Model file for the job. Use its own axes, mm. A direction names the side the tool comes from. Coordinates: 2 decimals unless noted, no trailing zeros. Order: outer loops, then holes, each group sorted by start corner. A loop starts at its lowest first (then second) coordinate and runs counter-clockwise, first axis right, second up. Notation, with made-up numbers: (26.5, -33) - (66.5, -33) arc R10 cw to (66.5, -29) - close; hole circle Ø5 at (-9, 47.25). An arc over 180 degrees is marked (long way). Put each result on its own line as item: value. Start each with the question number.
```python
from build123d import *

# Parameters (mm, degrees)
ESQUISSE1_R      = 5
EXTRUSION1_DEPTH = 3
ESQUISSE3_R      = 2
EXTRUSION3_DEPTH = 2
ESQUISSE4_R      = 5
EXTRUSION4_DEPTH = 1
ESQUISSE5_W      = 6
ESQUISSE5_H      = 12
EXTRUSION5_DEPTH = 10
ESQUISSE6_W      = 3
ESQUISSE6_H      = 2
EXTRUSION6_DEPTH = 5
ESQUISSE2_R      = 2.5
EXTRUSION7_DEPTH = 2


with BuildPart() as part:
    # Esquisse1 → Extrusion1 (new body)
    with BuildSketch(Plane(origin=(0, 0, 0), x_dir=(1, 0, 0), z_dir=(0, 1, 0))):
        Circle(ESQUISSE1_R)
    extrude(amount=EXTRUSION1_DEPTH)

    # Esquisse3 → Extrusion3 (add)
    with BuildSketch(Plane.XZ):
        Circle(ESQUISSE3_R)
    extrude(amount=EXTRUSION3_DEPTH)

    # Esquisse4 → Extrusion4 (add)
    with BuildSketch(Plane.XZ.offset(2)):
        Circle(ESQUISSE4_R)
    extrude(amount=EXTRUSION4_DEPTH)

    # Esquisse5 → Extrusion5 (add)
    with BuildSketch(Plane.XZ.offset(3)):
        Rectangle(ESQUISSE5_W, ESQUISSE5_H)
    extrude(amount=EXTRUSION5_DEPTH)

    # Esquisse6 → Extrusion6 (add)
    with BuildSketch(Plane.XZ.offset(13)):
        with Locations((0, 4)):
            Rectangle(ESQUISSE6_W, ESQUISSE6_H)
        Rectangle(ESQUISSE6_W, ESQUISSE6_H)
        with Locations((0, -4)):
            Rectangle(ESQUISSE6_W, ESQUISSE6_H)
    extrude(amount=EXTRUSION6_DEPTH)

    # Esquisse2 → Extrusion7 (cut)
    with BuildSketch(Plane(origin=(0, 3, 0), x_dir=(-1, 0, 0), z_dir=(0, 1, 0))):
        Circle(ESQUISSE2_R)
    extrude(amount=-EXTRUSION7_DEPTH, mode=Mode.SUBTRACT)


solid = part.part
```
Item 1: Wall check: line 1 along Z through (x, y) = (0, 2.35); line 2 along Y through (x, z) = (-2, -2); line 3 along Y through (x, z) = (-0.5, 4.75). Give the ranges that are in metal, low to high.
Item 2: Flat gauge pins, fed straight in: pin 1 Ø3.5 at (x, y) = (0.5, -16.5) entering from +Z; pin 2 Ø6 at (y, z) = (-13, -1.5) entering from +X; pin 3 Ø2 at (y, z) = (-16.5, -4) entering from +X. Where does each tip first touch, or does it go through?
Item 3: Pull direction Z, two halves, no side cores. Call faces 1 (the face through (-1.5, -15, 0)), 2 (the face through (0, -13, 1.4)), 3 (the face through (0, -15, 5)): pulls with the +Z half, pulls with the -Z half, needs draft (parallel to the pull), parting line crosses it, or undercut.
Item 4: Slice it at C-C, the plane z = 0. Give the cut face in (x, y), plus the area to 3 significant figures.
Item 5: 3-axis set-ups, long thin cutter, end or side, ignore diameter. For faces 4 (the face through (-4, -3, 0)), 5 (the face through (-1.08, 1.48, 4.88)), 6 (the face through (0, -15, -5)), 7 (the face through (-0.1, -2, -2.2)), 8 (the face through (4, -3, 0)): which of +Z, -Z, +X, -X, +Y, -Y reach the whole face in a straight line?
Item 6: Slice it at D-D, the plane x = -2.25. Give the cut face in (y, z), plus the area to 3 significant figures.
Item 7: Slice it at A-A, the plane y = -15.5. Give the cut face in (x, z), plus the area to 3 significant figures.
Here are the results:
1. line 1: z = -5 to -2.5, 2.5 to 5
1. line 2: y = -13 to -2, 0 to 3
1. line 3: y = -18 to -2, 0 to 3
2. pin 1: stops at z = 5
2. pin 2: stops at x = 3
2. pin 3: stops at x = 1.5
3. face 1: needs draft
3. face 2: undercut
3. face 3: pulls with the +Z half
4. outline: (-5, -3) - (-3, -3) - (-3, -13) - (-1.5, -13) - (-1.5, -18) - (1.5, -18) - (1.5, -13) - (3, -13) - (3, -3) - (5, -3) - (5, -2) - (2, -2) - (2, 0) - (5, 0) - (5, 3) - (2.5, 3) - (2.5, 1) - (-2.5, 1) - (-2.5, 3) - (-5, 3) - (-5, 0) - (-2, 0) - (-2, -2) - (-5, -2) - close
4. area: 113 mm^2
5. face 4: +Z, -Z, -X, -Y
5. face 5: +Y
5. face 6: -Z, +X, -X, -Y
5. face 7: none
5. face 8: +Z, -Z, +X, -Y
6. outline: (-13, -6) - (-3, -6) - (-3, -4.47) - (-2, -4.47) - (-2, 4.47) - (-3, 4.47) - (-3, 6) - (-13, 6) - close; (0, -4.47) - (3, -4.47) - (3, -1.09) - (1, -1.09) - (1, 1.09) - (3, 1.09) - (3, 4.47) - (0, 4.47) - close
6. area: 151 mm^2
7. outline: (-1.5, -5) - (1.5, -5) - (1.5, -3) - (-1.5, -3) - close; (-1.5, -1) - (1.5, -1) - (1.5, 1) - (-1.5, 1) - close; (-1.5, 3) - (1.5, 3) - (1.5, 5) - (-1.5, 5) - close
7. area: 18.0 mm^2
